```python
from build123d import *

# Parameters (mm, degrees)
EXTRUDE_1_DEPTH     = 20
SKETCH_4_R          = 2
CUT_EXTRUDE_1_DEPTH = 8
CUT_EXTRUDE_2_REACH = 48.989
SKETCH_5_R          = 2
SKETCH_6_R          = 3.5
CUT_EXTRUDE_3_DEPTH = 2
CUT_EXTRUDE_4_DEPTH = 3


with BuildPart() as part:
    # Эскиз1 → Бобышка-Вытянуть1 (new body)
    with BuildSketch(Plane.XY):
        with BuildLine():
            Line((-22, 0), (20, 0))
            Line((20, 0), (20, 8))
            Line((20, 8), (10, 8))
            Line((10, 8), (10, 28))
            Line((10, 28), (0.5, 28))
            Line((0.5, 28), (0.5, 19.979130372))
            ThreePointArc((0.5, 19.979130372), (0, 8), (-0.5, 19.979130372))
            Line((-0.5, 19.979130372), (-0.5, 28))
            Line((-0.5, 28), (-10, 28))
            Line((-10, 28), (-10, 8))
            Line((-10, 8), (-22, 8))
            Line((-22, 8), (-22, 0))
        make_face()
    extrude(amount=EXTRUDE_1_DEPTH)

    # Эскиз4 → Вырез-Вытянуть1 (cut)
    with BuildSketch(Plane(origin=(0, 8, 0), x_dir=(1, 0, 0), z_dir=(0, 1, 0))):
        with Locations(Location((15, -10, 0), (0, 0, 180))):
            Circle(SKETCH_4_R)
        with Locations(Location((-17, -10, 0), (0, 0, 180))):
            Circle(SKETCH_4_R)
    extrude(amount=-CUT_EXTRUDE_1_DEPTH, mode=Mode.SUBTRACT)

    # Вырез-Вытянуть2: up to this face of the body (flat: up to its plane)
    cut_extrude_2_end = Plane(part.part.faces().sort_by_distance((-10, 18, 10))[0])
    # Эскиз5 → Вырез-Вытянуть2 (cut, up to the picked face)
    with BuildSketch(Plane(origin=(10, 0, 0), x_dir=(0, 0, -1), z_dir=(1, 0, 0)), mode=Mode.PRIVATE) as cut_extrude_2_sk1:
        with Locations((-10, 24)):
            Circle(SKETCH_5_R)
    cut_extrude_2_tool1 = split(extrude(cut_extrude_2_sk1.sketch, amount=-CUT_EXTRUDE_2_REACH, mode=Mode.PRIVATE), bisect_by=cut_extrude_2_end, keep=Keep.BOTH, mode=Mode.PRIVATE)
    add(cut_extrude_2_tool1.solids().sort_by(Axis((10, 24, 10), (-1, 0, 0)))[0], mode=Mode.SUBTRACT)

    # Эскиз6 → Вырез-Вытянуть3 (cut)
    with BuildSketch(Plane(origin=(10, 0, 0), x_dir=(0, 0, -1), z_dir=(1, 0, 0))):
        with Locations((-10, 24)):
            Circle(SKETCH_6_R)
    extrude(amount=-CUT_EXTRUDE_3_DEPTH, mode=Mode.SUBTRACT)

    # Эскиз7 → Вырез-Вытянуть4 (cut)
    with BuildSketch(Plane.ZY.offset(10)):
        Polygon((14.041451884, 24), (12.020725942, 27.5), (7.979274058, 27.5), (5.958548116, 24), (7.979274058, 20.5), (12.020725942, 20.5), align=None)
    extrude(amount=-CUT_EXTRUDE_4_DEPTH, mode=Mode.SUBTRACT)


solid = part.part
```
The model under review builds one solid part; all positions refer to its coordinate system, in mm. A direction names the side the tool comes from. Round coordinates to 2 decimals unless told otherwise and drop trailing zeros. Loops run counter-clockwise (first coordinate to the right, second up) from the corner with the lowest first, then second, coordinate; pieces in that order, holes last. Notation, with made-up numbers: (20, 18.25) -> (48, 18.25) arc R11 ccw to (48, 26.25) -> close; hole circle Ø1 at (-11.5, 86). An arc over 180 degrees is marked (long way). Answer as a JSON object with one key per item and string values. Group by question number.
1) We need section A-A on y = 14. Write out the cut boundary in (x, z).
2) We need section C-C on x = -17. Write out the cut boundary in (y, z).
3) We need section D-D on y = 2.25. Write out the cut boundary in (x, z), then the cut area to 3 significant figures.
4) For pin 1 Ø6 at (x, z) = (-16.5, 10.5) entering from -Y; pin 2 Ø9 at (y, z) = (23, 5) entering from +X; pin 3 Ø4.5 at (y, z) = (24, 10) entering from +X; pin 4 Ø11 at (y, z) = (24, 10) entering from -X, all flat-tipped, find the tip position at first contact; note any pin that passes through.
5) Mouldability with a two-part tool opening along X and no side actions: class faces 5 (the face through (-10, 18, 10)), 6 (the face through (-8.5, 25.8, 7)), 7 (the face through (-15.526, 4.056, 11.352)), 8 (the face through (8, 22, 8)) as released by +X, released by -X, zero draft, split by the parting line, or undercut.
6) We need section B-B on x = 3. Write out the cut boundary in (y, z).
7) For faces 1 (the face through (9.01, 27.47, 10.46)), 2 (the face through (-8.521, 25.726, 13.045)), 3 (the face through (0.5, 24, 7.6)), 4 (the face through (10, 18, 10)), list the 3-axis set-ups (+Z, -Z, +X, -X, +Y, -Y) from which the entire face can be reached by the end or side of a thin tool; tool diameter is ignored.
8) For line 1 (X direction, y = 14, z = 13); line 2 (X direction, y = 21.5, z = 7.5); line 3 (Y direction, x = 8.55, z = 10), list the stretches that pass through material, from the lowest coordinate up. Write a range as [from, to].
Result set:
{
 "1": {"outline": "(-10, 0) -> (-6, 0) -> (-6, 20) -> (-10, 20) -> close; (6, 0) -> (10, 0) -> (10, 20) -> (6, 20) -> close"},
 "2": {"outline": "(0, 0) -> (8, 0) -> (8, 8) -> (0, 8) -> close; (0, 12) -> (8, 12) -> (8, 20) -> (0, 20) -> close"},
 "3": {"outline": "(-22, 0) -> (20, 0) -> (20, 20) -> (-22, 20) -> close; hole circle Ø4 at (-17, 10); hole circle Ø4 at (15, 10)", "area": "815 mm²"},
 "4": {"pin 1": "y = 0", "pin 2": "x = 10", "pin 3": "x = 8", "pin 4": "x = -10"},
 "5": {"face 5": "released by -X", "face 6": "zero draft", "face 7": "undercut", "face 8": "released by +X"},
 "6": {"outline": "(0, 0) -> (8.8, 0) -> (8.8, 20) -> (0, 20) -> close; (19.2, 0) -> (28, 0) -> (28, 20) -> (19.2, 20) -> close; hole circle Ø4 at (24, 10)"},
 "7": {"face 1": "+X", "face 2": "-X", "face 3": "+Z, -Z, +Y", "face 4": "+Z, -Z, +X, +Y"},
 "8": {"line 1": "[-10, -6], [6, 10]", "line 2": "[-7, -0.5], [0.5, 10]", "line 3": "[0, 20.5], [27.5, 28]"}
}
